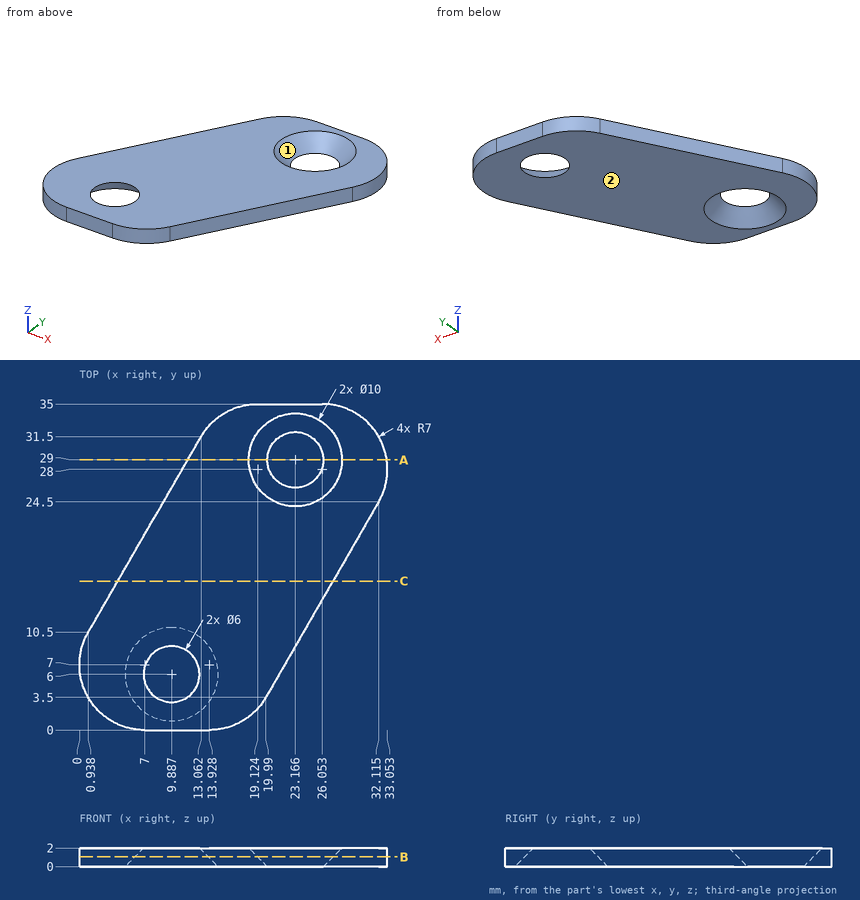
The drawing under review shows one solid part. Ordinate dimensions are in mm from its lowest x, y, z. Coordinates: 2 decimals unless noted, no trailing zeros. Order: outer loops, then holes, each group sorted by start corner. A loop starts at its lowest first (then second) coordinate and runs counter-clockwise, first axis right, second up. Notation, with made-up numbers: (23, -30.5) -> (37, -30.5) arc R21 cw to (37, 3.5) -> close; hole circle Ø8 at (-22.5, 31.25). An arc over 180 degrees is marked (long way). Return JSON: item names as keys, results as strings.
1. For line 1 (X direction, y = 26, z = 1.8) (1 decimal); line 2 (Y direction, x = 21.5, z = 0.15) (1 decimal); line 3 (Y direction, x = 10.5, z = 1.45) (1 decimal), list the stretches that pass through material, from the lowest coordinate up. Write a range as from..to.
Answer block:
{"line 1": "9.9..19.4, 26.9..32.8", "line 2": "6.1..26.3, 31.7..35", "line 3": "0..2.5, 9.5..27.1"}
2. The part is to be moulded in two halves that separate along Y. For the marked faces 1 and 2, say which applies: +Y half, -Y half, draft (parallel to the pull), parting line (faces both ways), or undercut.
Answer block:
{"face 1": "undercut", "face 2": "draft"}
3. We need section C-C on y = 16. Write out the cut boundary in (x, z).
Answer block:
{"outline": "(4.11, 0) -> (27.21, 0) -> (27.21, 2) -> (4.11, 2) -> close"}
4. We need section B-B on z = 1.05. State how many separate pieces and enclosed holes the cut face has, and give its area (3 significant figures).
Answer block:
{"separate pieces": "1", "enclosed holes": "2", "area": "635 mm²"}
5. We need section A-A on y = 29. Write out the cut boundary in (x, z) (1 decimal).
Answer block:
{"outline": "(11.6, 0) -> (20.2, 0) -> (18.2, 2) -> (11.6, 2) -> close; (26.2, 0) -> (33, 0) -> (33, 2) -> (28.2, 2) -> close"}
